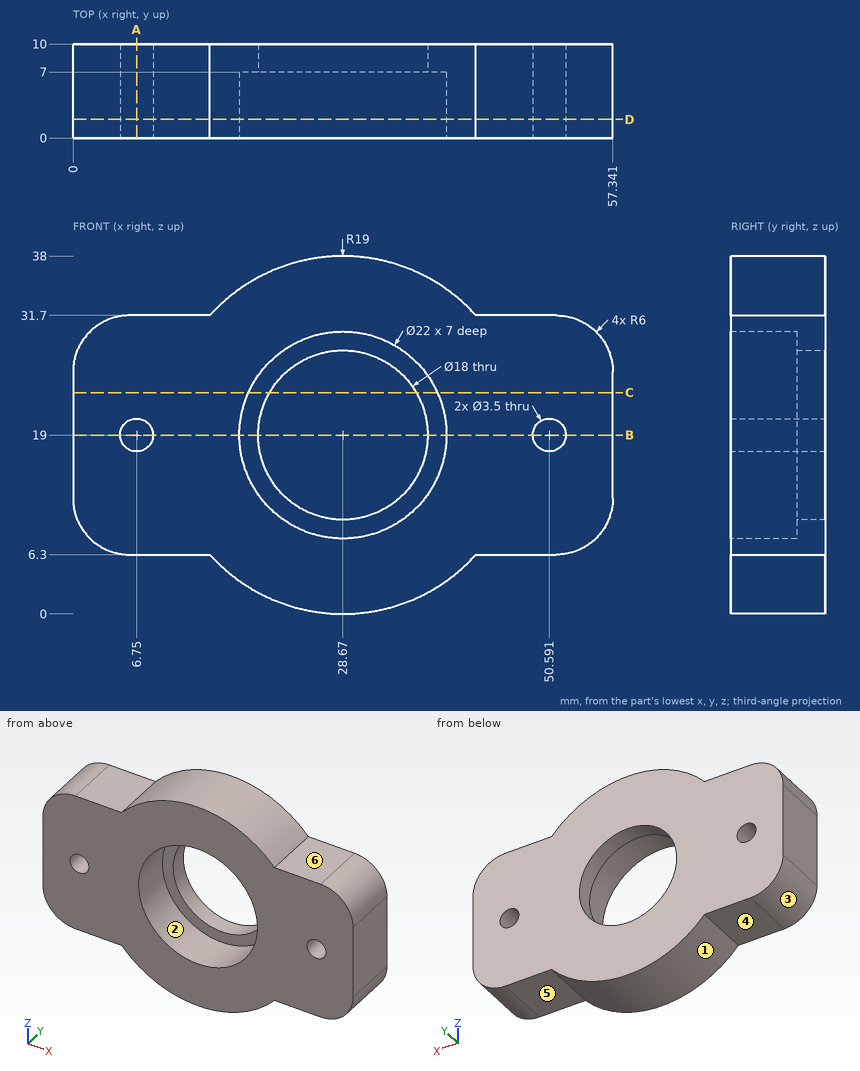
Job drawing, mm, ordinate dimensions from the low corner. One solid piece. A direction names the side the tool comes from. Round coordinates to 2 decimals unless told otherwise and drop trailing zeros. Write each loop counter-clockwise with the first axis right and the second up, starting at its lowest first coordinate (ties: lowest second). Pieces come first, ordered by that corner, then holes.
1) Pin check, flat tips, straight feed: pin 1 (6 mm diameter, centred on x = 34, z = 15, fed in from -Y); pin 2 (6 mm diameter, centred on x = 51, y = 3, fed in from +Z); pin 3 (4.5 mm diameter, centred on x = 10.5, y = 4, fed in from -Z). Stop position of each tip, or through.
2) Mould opens along X. For the marked faces 1, 2 and 3 say: +X half, -X half, draft (parallel to the pull), parting line (faces both ways), or undercut.
3) Band-saw the part on C-C, the plane z = 23.5. List the corners of the cut face in (x, y) (1 decimal), and give its area (3 significant figures).
4) 3-axis set-ups, long thin cutter, end or side, ignore diameter. For the marked faces 4, 5 and 6: which of +Z, -Z, +X, -X, +Y, -Y reach the whole face in a straight line?
5) Band-saw the part on A-A, the plane x = 6.75. List the corners of the cut face in (y, z), and give its area (3 significant figures).
6) Band-saw the part on D-D, the plane y = 2. List the corners of the cut face in (x, z).
7) Drill centre lines: probe 1 along X at (y, z) = (9.35, 19); probe 2 along X at (y, z) = (3.25, 19); probe 3 along Z at (x, y) = (48, 1). Where is each one in solid material? Low to high.
8) Band-saw the part on B-B, the plane z = 19. List the corners of the cut face in (x, y).
Ans:
1. pin 1: stops at y = 7
1. pin 2: stops at z = 31.7
1. pin 3: stops at z = 6.3
2. face 1: parting line
2. face 2: undercut
2. face 3: -X half
3. outline: (0, 0) - (18.6, 0) - (18.6, 7) - (20.9, 7) - (20.9, 10) - (0, 10) - close; (36.5, 7) - (38.7, 7) - (38.7, 0) - (57.3, 0) - (57.3, 10) - (36.5, 10) - close
3. area: 386 mm2
4. face 4: -Z, -X, +Y, -Y
4. face 5: -Z, +X, +Y, -Y
4. face 6: +Z, +X, +Y, -Y
5. outline: (0, 6.3) - (10, 6.3) - (10, 17.25) - (0, 17.25) - close; (0, 20.75) - (10, 20.75) - (10, 31.7) - (0, 31.7) - close
5. area: 219 mm2
6. outline: (0, 12.3) arc R6 ccw to (6, 6.3) - (14.54, 6.3) arc R19 ccw to (42.8, 6.3) - (51.34, 6.3) arc R6 ccw to (57.34, 12.3) - (57.34, 25.7) arc R6 ccw to (51.34, 31.7) - (42.8, 31.7) arc R19 ccw to (14.54, 31.7) - (6, 31.7) arc R6 ccw to (0, 25.7) - close; hole circle Ø3.5 at (6.75, 19); hole circle Ø22 at (28.67, 19); hole circle Ø3.5 at (50.59, 19)
7. probe 1: x = 0 to 5, 8.5 to 19.67, 37.67 to 48.84, 52.34 to 57.34
7. probe 2: x = 0 to 5, 8.5 to 17.67, 39.67 to 48.84, 52.34 to 57.34
7. probe 3: z = 6.3 to 31.7
8. outline: (0, 0) - (5, 0) - (5, 10) - (0, 10) - close; (8.5, 0) - (17.67, 0) - (17.67, 7) - (19.67, 7) - (19.67, 10) - (8.5, 10) - close; (37.67, 7) - (39.67, 7) - (39.67, 0) - (48.84, 0) - (48.84, 10) - (37.67, 10) - close; (52.34, 0) - (57.34, 0) - (57.34, 10) - (52.34, 10) - close
